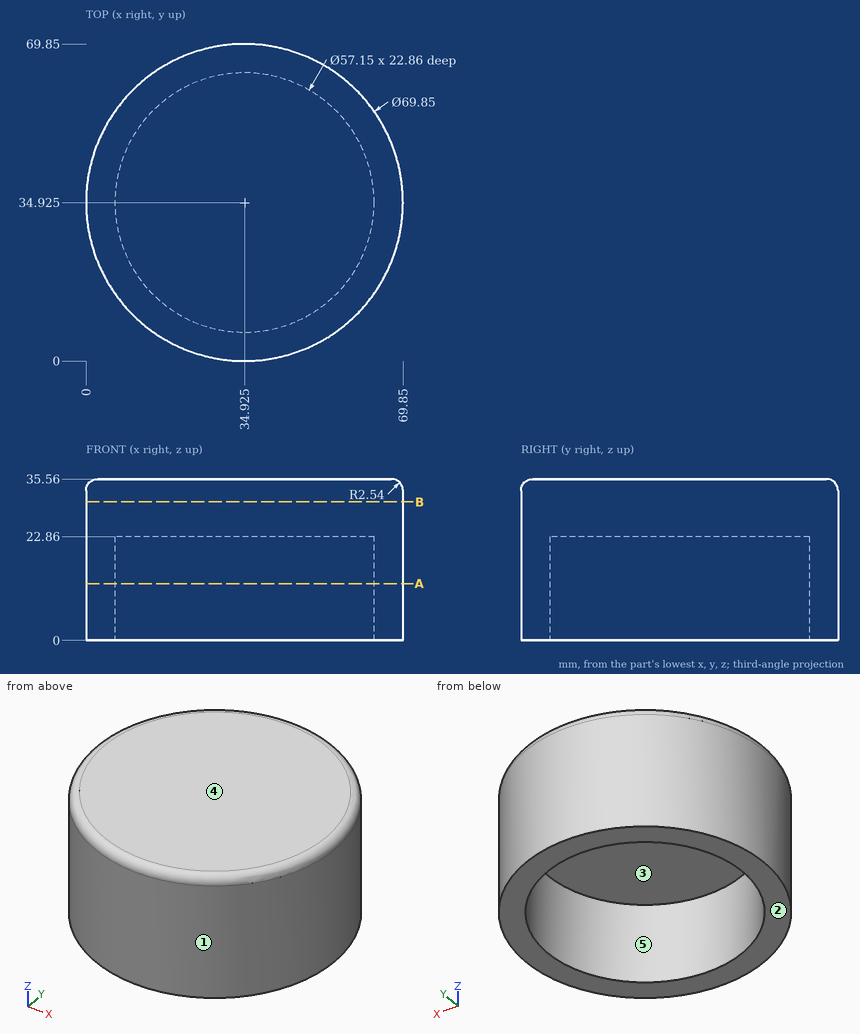
Part print with two shaded views. Sizes in mm from the minimum x, y, z corner. A direction names the side the tool comes from. Coordinates: 2 decimals unless noted, no trailing zeros. Loops run counter-clockwise (first coordinate to the right, second up) from the corner with the lowest first, then second, coordinate; pieces in that order, holes last. Notation, with made-up numbers: (59, 8.5) - (101, 8.5) arc R14 cw to (101, 28.5) - close; hole circle Ø5 at (5, -3). An arc over 180 degrees is marked (long way). Write each question's results on one line, items separated by ' | '. Start each with the question number.
Q1. Slice it at B-B on z = 30.5. Give the cut face in (x, y) (3 decimals).
Q2. Slice it at A-A on z = 12.5. Give the cut face in (x, y) (3 decimals), and give its area (3 significant figures).
Q3. Two-plate mould, pull along Y, no slides. Class the marked faces 1, 2 and 3: +Y half, -Y half, draft (parallel to the pull), parting line (faces both ways), or undercut.
Q4. Drop flat-ended pins along their axis: pin 1 Ø6 at (x, z) = (21.5, 22) entering from -Y; pin 2 Ø4 at (y, z) = (47.5, 31.5) entering from -X; pin 3 Ø8 at (y, z) = (27.5, 12) entering from -X. Give the stop position or say it passes through.
Q5. Probe line 1 along Z through (x, y) = (42, 41); line 2 along Y through (x, z) = (41, 19.5); line 3 along X through (y, z) = (9.5, 7). List the from-to ranges inside material, lowest first.
Q6. Which spindle directions (+Z, -Z, +X, -X, +Y, -Y) get a long thin tool onto all of the face, cutting with end or side? Do the marked faces 4 and 5. Say none if no direction does.
Answer:
1) outline: circle Ø69.85 at (34.925, 34.925)
2) outline: circle Ø69.85 at (34.925, 34.925); hole circle Ø57.15 at (34.925, 34.925) | area: 1,270 mm2
3) face 1: parting line | face 2: draft | face 3: undercut
4) pin 1: stops at y = 1.59 | pin 2: stops at x = 1.64 | pin 3: stops at x = 0.17
5) line 1: z = 22.86 to 35.56 | line 2: y = 0.53 to 7, 62.85 to 69.32 | line 3: x = 10.98 to 21.88, 47.97 to 58.87
6) face 4: +Z, +X, -X, +Y, -Y | face 5: -Z
